```python
from build123d import *

# Parameters (mm, degrees)
BOSS_EXTRUDE1_DEPTH = 122
BOSS_EXTRUDE2_DEPTH = 80
CHAMFER2_SIZE       = 20


with BuildPart() as part:
    # Sketch1 → Boss-Extrude1 (new body)
    with BuildSketch(Plane.XY):
        with BuildLine():
            Line((-24.448977817, 50.585997889), (-24.448977817, 47.607417283))
            Line((-24.448977817, 47.607417283), (-31.698977817, 47.607417283))
            Line((-31.698977817, 47.607417283), (-31.698977817, 34.416624517))
            ThreePointArc((-31.698977817, 34.416624517), (-44.606827003, 13.925447751), (-40.708122297, -9.976455887))
            Line((-40.708122297, -9.976455887), (-31.917393168, -24.877445372))
            Line((-31.917393168, -24.877445372), (-34.51546938, -26.377445372))
            Line((-34.51546938, -26.377445372), (-38.01546938, -20.315267546))
            Line((-38.01546938, -20.315267546), (-41.046558293, -22.065267546))
            Line((-41.046558293, -22.065267546), (-38.546558293, -26.395394565))
            Line((-38.546558293, -26.395394565), (-41.144634504, -27.895394565))
            Line((-41.144634504, -27.895394565), (-44.144634504, -22.699242142))
            ThreePointArc((-44.144634504, -22.699242142), (-44.344435349, -21.181604052), (-43.412583697, -19.967191335))
            Line((-43.412583697, -19.967191335), (-41.388249315, -18.798441335))
            ThreePointArc((-41.388249315, -18.798441335), (-40.456397663, -17.584028617), (-40.656198508, -16.066390527))
            Line((-40.656198508, -16.066390527), (-43.306198508, -11.476455887))
            ThreePointArc((-43.306198508, -11.476455887), (-47.768566234, 13.330532327), (-35.392400045, 35.287988929))
            ThreePointArc((-35.392400045, 35.287988929), (-34.880578034, 35.969486614), (-34.698977817, 36.802206392))
            Line((-34.698977817, 36.802206392), (-34.698977817, 51.585997889))
            ThreePointArc((-34.698977817, 51.585997889), (-34.113191379, 53.000211451), (-32.698977817, 53.585997889))
            Line((-32.698977817, 53.585997889), (-16.448977817, 53.585997889))
            Line((-16.448977817, 53.585997889), (-16.448977817, 50.585997889))
            Line((-16.448977817, 50.585997889), (-24.448977817, 50.585997889))
        make_face()
    extrude(amount=BOSS_EXTRUDE1_DEPTH)

    # Sketch3 → Boss-Extrude2 (add)
    with BuildSketch(Plane.XY.offset(122)):
        Polygon((-31.698977817, 41.085997889), (-16.448977817, 41.085997889), (-16.448977817, 44.085997889), (-24.448977817, 44.085997889), (-24.448977817, 47.607417283), (-31.698977817, 47.607417283), align=None)
    extrude(amount=-BOSS_EXTRUDE2_DEPTH)

    # Chamfer2
    # the kernel refuses this chamfer: 20 mm, written as the material it adds along each edge
    with BuildSketch(Plane(origin=(-31.698977817, 47.607417283, 42), x_dir=(-0.02749587661058649, 0, -0.9996219169112968), z_dir=(0, -1, 0))) as chamfer2_piece_1_section:
        Polygon((CHAMFER2_SIZE * 0.999621916911, CHAMFER2_SIZE * 0.0274958766106), (-CHAMFER2_SIZE * 0.0274958766106, CHAMFER2_SIZE * 0.999621916911), (0, 0), align=None)
    chamfer2_piece_1 = extrude(amount=6.521419395, mode=Mode.PRIVATE)
    chamfer2_piece_1 = split(chamfer2_piece_1, bisect_by=Plane(origin=(-24.448977817, 45.846707586, 33.55788947), z_dir=(-1, 0, 0)), keep=Keep.TOP, mode=Mode.PRIVATE)
    chamfer2_piece_1 = split(chamfer2_piece_1, bisect_by=Plane(origin=(-28.61775968, 44.085997889, 33.55788947), z_dir=(0, 1, 0)), keep=Keep.TOP, mode=Mode.PRIVATE)
    add(chamfer2_piece_1)
    with BuildSketch(Plane(origin=(-31.698977817, 47.607417283, 42), x_dir=(-0.02749587661058649, 0, -0.9996219169112968), z_dir=(0, -1, 0))) as chamfer2_piece_2_section:
        Polygon((CHAMFER2_SIZE * 0.999621916911, CHAMFER2_SIZE * 0.0274958766106), (-CHAMFER2_SIZE * 0.0274958766106, CHAMFER2_SIZE * 0.999621916911), (0, 0), align=None)
    chamfer2_piece_2 = extrude(amount=6.521419395, mode=Mode.PRIVATE)
    chamfer2_piece_2 = split(chamfer2_piece_2, bisect_by=Plane(origin=(-24.448977817, 42.585997889, 33.55788947), z_dir=(-1, 0, 0)), keep=Keep.TOP, mode=Mode.PRIVATE)
    chamfer2_piece_2 = split(chamfer2_piece_2, bisect_by=Plane(origin=(-28.61775968, 44.085997889, 33.55788947), z_dir=(0, -1, 0)), keep=Keep.TOP, mode=Mode.PRIVATE)
    add(chamfer2_piece_2)
    with BuildSketch(Plane(origin=(-31.698977817, 47.607417283, 42), x_dir=(-0.02749587661058649, 0, -0.9996219169112968), z_dir=(0, -1, 0))) as chamfer2_piece_3_section:
        Polygon((CHAMFER2_SIZE * 0.999621916911, CHAMFER2_SIZE * 0.0274958766106), (-CHAMFER2_SIZE * 0.0274958766106, CHAMFER2_SIZE * 0.999621916911), (0, 0), align=None)
    chamfer2_piece_3 = extrude(amount=6.521419395, mode=Mode.PRIVATE)
    chamfer2_piece_3 = split(chamfer2_piece_3, bisect_by=Plane(origin=(-24.448977817, 42.585997889, 37.556915733), z_dir=(1, 0, 0)), keep=Keep.TOP, mode=Mode.PRIVATE)
    chamfer2_piece_3 = split(chamfer2_piece_3, bisect_by=Plane(origin=(-16.448977817, 42.585997889, 37.556915733), z_dir=(-1, 0, 0)), keep=Keep.TOP, mode=Mode.PRIVATE)
    chamfer2_piece_3 = split(chamfer2_piece_3, bisect_by=Plane(origin=(-21.010172904, 44.085997889, 37.556915733), z_dir=(0, -1, 0)), keep=Keep.TOP, mode=Mode.PRIVATE)
    add(chamfer2_piece_3)


solid = part.part
```
Work out the finished part from the listing and answer in its coordinate system (mm). A direction names the side the tool comes from. Coordinates: 2 decimals unless noted, no trailing zeros. Loops run counter-clockwise (first coordinate to the right, second up) from the corner with the lowest first, then second, coordinate; pieces in that order, holes last. Notation, with made-up numbers: (84.5, -12) -> (143.5, -12) arc R8 ccw to (143.5, -8) -> close; hole circle Ø9 at (84.5, 33.5). An arc over 180 degrees is marked (long way). Answer as CSV lines item,"result".
Q1. Find the intervals of material crossed by probe 1 along Y at (x, z) = (-39.5, 87.5); probe 2 along Y at (x, z) = (-22, 84); probe 3 along Y at (x, z) = (-29, 6), in increasing order.
Findings:
probe 1,"y = -26.95 to -24.74, -21.17 to -12.02, 26.16 to 31.14"
probe 2,"y = 41.09 to 44.09, 50.59 to 53.59"
probe 3,"y = 47.61 to 53.59"
Q2. For a pull along X with two mould halves and no side action, classify faces 6 (the face through (-41.963, -13.804, 60.146)), 7 (the face through (-44.536, 14.265, 60.146)), 8 (the face through (-39.814, -24.2, 60.146)), 9 (the face through (-20, 44.086, 76)) as +X half, -X half, draft (parallel to the pull), parting line (faces both ways), or undercut.
Findings:
face 6,"-X half"
face 7,"+X half"
face 8,"undercut"
face 9,"draft"
Q3. The part is cut by section D-D on y = 13. Write down the section's boundary in (x, z), and give its area (3 significant figures).
Findings:
outline,"(-47.82, 0) -> (-44.78, 0) -> (-44.78, 122) -> (-47.82, 122) -> close"
area,"371 mm²"
Q4. The part is cut by section A-A on x = -21.5. Write down the section's boundary in (y, z), and give its area (3 significant figures).
Findings:
outline,"(41.09, 32.2) -> (44.09, 32.2) -> (44.09, 122) -> (41.09, 122) -> close; (50.59, 0) -> (53.59, 0) -> (53.59, 122) -> (50.59, 122) -> close"
area,"635 mm²"
Q5. Each of these flat-tipped pins is pushed along its axis until it touches: pin 1 (3.5 mm diameter, centred on x = -28.5, z = 15, fed in from -Y); pin 2 (1.5 mm diameter, centred on y = 5.5, z = 82, fed in from -X); pin 3 (2 mm diameter, centred on x = -22, z = 83, fed in from -Y). Where does it stop, or does it pass through?
Findings:
pin 1,"stops at y = 47.61"
pin 2,"stops at x = -48.28"
pin 3,"stops at y = 41.09"
Q6. The part is cut by section B-B on z = 100. Write down the section's boundary in (x, y).
Findings:
outline,"(-44.14, -22.7) -> (-41.14, -27.9) -> (-38.55, -26.4) -> (-41.05, -22.07) -> (-38.02, -20.32) -> (-34.52, -26.38) -> (-31.92, -24.88) -> (-40.71, -9.98) arc R34.2 cw to (-31.7, 34.42) -> (-31.7, 41.09) -> (-16.45, 41.09) -> (-16.45, 44.09) -> (-24.45, 44.09) -> (-24.45, 50.59) -> (-16.45, 50.59) -> (-16.45, 53.59) -> (-32.7, 53.59) arc R2 ccw to (-34.7, 51.59) -> (-34.7, 36.8) arc R2 cw to (-35.39, 35.29) arc R37.2 ccw to (-43.31, -11.48) -> (-40.66, -16.07) arc R2 cw to (-41.39, -18.8) -> (-43.41, -19.97) arc R2 ccw to start"
Q7. A tool of negligible diameter and unlimited length cuts with its end or side. For faces 1 (the face through (-34.699, 44, 60)), 2 (the face through (-40.462, -17.605, 60.146)), 3 (the face through (-36.374, -17.323, 60.146)), 4 (the face through (-24, 41.086, 73)), 5 (the face through (-31.699, 38, 47)), from which of +Z, -Z, +X, -X, +Y, -Y can it reach the whole face along a straight path? Write none if from no direction.
Findings:
face 1,"+Z, -Z, -X, +Y"
face 2,"+Z, -Z, -X"
face 3,"+Z, -Z, +X"
face 4,"+Z, -Z, +X, -Y"
face 5,"-Z, +X, -Y"
Q8. The part is cut by section C-C on x = -27.5. Write down the section's boundary in (y, z), and give its area (3 significant figures).
Findings:
outline,"(41.09, 26.2) -> (47.61, 26.2) -> (47.61, 0) -> (53.59, 0) -> (53.59, 122) -> (41.09, 122) -> close"
area,"1,350 mm²"
